from build123d import *

# Parameters (mm, degrees)
F1_DEPTH = 2
F2_D     = 6
F3_R     = 5


with BuildPart() as f1:
    # F0 (on Top) → F1 (new body)
    with BuildSketch(Plane.XY):
        with BuildLine():
            Line((0, 31.5), (-98.5, 31.5))
            Line((-98.5, 31.5), (-98.5, -31.5))
            Line((-98.5, -31.5), (0, -31.5))
            ThreePointArc((0, -31.5), (31.5, 0), (0, 31.5))
        make_face()
        with BuildLine():
            Line((-9.25, -5), (-89.25, -5))
            ThreePointArc((-89.25, -5), (-94.25, 0), (-89.25, 5))
            Line((-89.25, 5), (-9.25, 5))
            ThreePointArc((-9.25, 5), (-4.25, 0), (-9.25, -5))
        make_face(mode=Mode.SUBTRACT)
    extrude(amount=F1_DEPTH)

    # F2 (through all)
    with Locations(Plane(origin=(0, 0, 0), x_dir=(1, 0, 0), z_dir=(0, 0, -1))):
        with Locations((-93.2, -26.7), (-93.2, 14.5), (-29.3, -26.7), (-29.3, 23.3), (11.5, 0)):
            Hole(F2_D / 2)

    # F3
    f3_edges = [f1.edges().sort_by_distance(p)[0] for p in [
        (-98.5, 31.5, 1),
        (-98.5, -31.5, 1),
    ]]
    fillet(f3_edges, radius=F3_R)


solid = f1.part
Part model, mm, in its own coordinate system. A direction names the side the tool comes from. Round coordinates to 2 decimals unless told otherwise and drop trailing zeros. Write each loop counter-clockwise with the first axis right and the second up, starting at its lowest first coordinate (ties: lowest second). Pieces come first, ordered by that corner, then holes. Notation, with made-up numbers: M 8,59.5 L 15,59.5 A21 cw 15,74.5 Z; hole C -10,-34 d9. An arc over 180 degrees is marked long. Return JSON: item names as keys, results as strings. Group by question number.
(1) Saw through at A-A on x = -50. Write the cut outline in (y, z), then the cut area to 3 significant figures.
(2) Drill centre lines: probe 1 along Y at (x, z) = (-29.3, 1.5); probe 2 along Y at (x, z) = (-24, 1.85); probe 3 along X at (y, z) = (29, 1.3). Where is each one in solid material? Low to high.
(3) Saw through at B-B on z = 0.8. Write the cut outline in (x, y).
(4) Saw through at D-D on y = 14. Write the cut outline in (x, z).
(5) Pin check, flat tip, straight feed: pin 1 Ø5.5 at (x, y) = (11.5, 0) entering from +Z. Stop position of the tip, or through.
(6) Saw through at C-C on y = -14.5. Write the cut outline in (x, z).
(7) Two-plate mould, pull along X, no slides. Class faces 3 (the face through (-34, -7, 0)), 4 (the face through (-26.3, -23.4, 1)), 5 (the face through (-97.07, -30, 1.01)): +X half, -X half, draft (parallel to the pull), parting line (faces both ways), or undercut.
(8) Which spindle directions (+Z, -Z, +X, -X, +Y, -Y) get a long thin tool onto all of the face, cutting with end or side? Do faces 1 (the face through (-94.25, -0.11, 0.99)), 2 (the face through (31.492, -0.693, 0.986)). Say none if no direction does.
Returned:
{
 "1": {"outline": "M -31.5,0 L -5,0 L -5,2 L -31.5,2 Z; M 5,0 L 31.5,0 L 31.5,2 L 5,2 Z", "area": "106 mm²"},
 "2": {"probe 1": "-31.5 to -26.3, -20.3 to -5, 5 to 23.7, 29.7 to 31.5", "probe 2": "-31.5 to -5, 5 to 31.5", "probe 3": "-97.83 to -95.13, -91.27 to -31.23, -27.37 to 12.3"},
 "3": {"outline": "M -98.5,-26.5 A5 ccw -93.5,-31.5 L 0,-31.5 A31.5 ccw 0,31.5 L -93.5,31.5 A5 ccw -98.5,26.5 Z; hole C -93.2,-14.5 d6; hole C -93.2,26.7 d6; hole M -89.25,-5 L -9.25,-5 A5 ccw -9.25,5 L -89.25,5 A5 ccw Z; hole C -29.3,-23.3 d6; hole C -29.3,26.7 d6; hole C 11.5,0 d6"},
 "4": {"outline": "M -98.5,0 L 28.22,0 L 28.22,2 L -98.5,2 Z"},
 "5": {"pin 1": "through"},
 "6": {"outline": "M -98.5,0 L -96.2,0 L -96.2,2 L -98.5,2 Z; M -90.2,0 L 27.96,0 L 27.96,2 L -90.2,2 Z"},
 "7": {"face 3": "draft", "face 4": "undercut", "face 5": "-X half"},
 "8": {"face 1": "+Z, -Z", "face 2": "+Z, -Z, +X"}
}
